from build123d import *
from build123d.topology import SkipClean

# Parameters (mm, degrees)
SKETCH_1_R               = 40
EXTRUDE_1_DEPTH          = 5
SKETCH_2_R               = 7.5
EXTRUDE_2_DEPTH          = 38
SKETCH_3_W               = 1.5
SKETCH_3_H               = 4.460741585
SKETCH_4_R               = 6
EXTRUDE_3_DEPTH          = 15
CHAMFER_1_SIZE           = 0.5
SKETCH_5_W               = 7.892485333
SKETCH_5_H               = 4
CUT_EXTRUDE_1_DEPTH      = 15
FILLET_1_R               = 2
EXTRUDE_START            = 33
SKETCH_6_R               = 40
SKETCH_6_R_2             = 30
EXTRUDE_4_DEPTH          = 33
PATTERN_CIRCULAR_1_COUNT = 4
CUT_EXTRUDE_2_DEPTH      = 33
PATTERN_CIRCULAR_2_COUNT = 2
PATTERN_CIRCULAR_2_ANGLE = 90
SKETCH_12_R              = 8.5
CUT_EXTRUDE_3_DEPTH      = 2
HOLE_WIZARD_M6_1_D       = 5
HOLE_WIZARD_M6_1_DEPTH   = 15
HOLE_WIZARD_M6_1_TIP     = 1.502151548
CUT_EXTRUDE_4_DEPTH      = 10
PATTERN_CIRCULAR_3_COUNT = 4
CHAMFER_2_SIZE           = 2
HOLE_WIZARD_M5_1_D       = 4.2
HOLE_WIZARD_M5_1_DEPTH   = 12.4
HOLE_WIZARD_M5_1_TIP     = 1.2618073


# Some blends are built 0.0001 mm under size
with BuildPart() as part:
    # 草图1 → 凸台-拉伸1 (new body)
    with BuildSketch(Plane.XY):
        with Locations((-62.277052722, 0)):
            Circle(SKETCH_1_R)
    extrude(amount=EXTRUDE_1_DEPTH)

    # 草图2 → 凸台-拉伸2 (add)
    with BuildSketch(Plane.XY.offset(5)):
        with Locations((-62.277052722, 0)):
            Circle(SKETCH_2_R)
    extrude(amount=EXTRUDE_2_DEPTH)

    # 草图3 → 切除-旋转1 (revolve, cut)
    with BuildSketch(Plane(origin=(0, 0, 0), x_dir=(0, 0, -1), z_dir=(0, -1, 0)), mode=Mode.PRIVATE) as cut_revolve_1_sk:
        with Locations((-40.75, -53.54668193)):
            Rectangle(SKETCH_3_W, SKETCH_3_H)
    revolve(cut_revolve_1_sk.sketch.rotate(Axis((-62.277052722, 0, 23.170133407), (0, 0, 1)), 180), axis=Axis((-62.277052722, 0, 23.170133407), (0, 0, 1)), mode=Mode.SUBTRACT)

    # 草图4 → 凸台-拉伸3 (add)
    with BuildSketch(Plane.XY.offset(43)):
        with Locations((-62.277052722, 0)):
            Circle(SKETCH_4_R)
    extrude(amount=EXTRUDE_3_DEPTH)

    # 倒角1
    chamfer_1_edges = [part.edges().sort_by_distance(p)[0] for p in [
        (-68.277052722, 0, 58),
        (-102.277052722, 0, 5),
        (-69.777052722, 0, 43),
    ]]
    chamfer(chamfer_1_edges, length=CHAMFER_1_SIZE)

    # 草图5 → 切除-拉伸1 (cut)
    with BuildSketch(Plane.XY.offset(58)):
        with Locations((-54.330810056, 0)):
            Rectangle(SKETCH_5_W, SKETCH_5_H)
    extrude(amount=-CUT_EXTRUDE_1_DEPTH, mode=Mode.SUBTRACT)

    # 圆角1
    fillet_1_edges = [part.edges().sort_by_distance(p)[0] for p in [
        (-57.448625597, -2, 43),
        (-57.448625597, 2, 43),
    ]]
    fillet(fillet_1_edges, radius=FILLET_1_R - 0.0001)  # a hair under: the kernel refuses the full size

    # 草图6 → 凸台-拉伸4 (add)
    with SkipClean():  # the faces are left unmerged after this step: merging them gives an invalid solid
        with BuildSketch(Plane(origin=(0, 0, 0), x_dir=(-1, 0, 0), z_dir=(0, 0, -1)).offset(EXTRUDE_START)):
            with Locations((62.277052722, 0)):
                Circle(SKETCH_6_R)
            with Locations((62.277052722, 0)):
                Circle(SKETCH_6_R_2, mode=Mode.SUBTRACT)
        extrude(amount=-EXTRUDE_4_DEPTH)

    # 草图9 → M8 螺纹孔1 (revolve, cut)
    with SkipClean():  # the faces are left unmerged after this step: merging them gives an invalid solid
        with BuildSketch(Plane(origin=(-97.277052722, 0, -33), x_dir=(0, 1, 0), z_dir=(1, 0, 0))):
            Polygon((0, 0), (0, 21.792926105), (3.4, 19.75), (3.4, 0), align=None)
        hole_wizard_m8_1 = revolve(axis=Axis((-97.277052722, 0, -39.35), (0, 0, 1)), mode=Mode.SUBTRACT)

    # 阵列(圆周)1: M8 螺纹孔1 ×4 about axis
    with SkipClean():  # the faces are left unmerged after this step: merging them gives an invalid solid
        pattern_circular_1_axis = Axis((-62.277052722, 0, 0), (0, 0, 1))
        for i in range(1, PATTERN_CIRCULAR_1_COUNT):
            add(hole_wizard_m8_1.rotate(pattern_circular_1_axis, i * 360 / PATTERN_CIRCULAR_1_COUNT), mode=Mode.SUBTRACT)

    # 草图11 → 切除-拉伸2 (cut)
    with SkipClean():  # the faces are left unmerged after this step: merging them gives an invalid solid
        with BuildSketch(Plane(origin=(0, 0, -33), x_dir=(-1, 0, 0), z_dir=(0, 0, -1))):
            Polygon((-32.267123115, 73.330972402), (135.608025124, -94.544175837), (156.82122856, -73.330972402), (-11.05391968, 94.544175837), align=None)
        cut_extrude_2 = extrude(amount=-CUT_EXTRUDE_2_DEPTH, mode=Mode.SUBTRACT)
    add(part.part.scale(1), mode=Mode.REPLACE)  # the faces are merged on a copy

    # 阵列(圆周)2: 切除-拉伸2 ×2 about axis
    pattern_circular_2_axis = Axis((-62.277052722, 0, -33), (0, 0, 1))
    for i in range(1, PATTERN_CIRCULAR_2_COUNT):
        add(cut_extrude_2.rotate(pattern_circular_2_axis, i * PATTERN_CIRCULAR_2_ANGLE / (PATTERN_CIRCULAR_2_COUNT - 1)), mode=Mode.SUBTRACT)

    # 草图12 → 切除-拉伸3 (cut)
    with BuildSketch(Plane(origin=(0, 0, 0), x_dir=(-1, 0, 0), z_dir=(0, 0, -1))):
        with Locations((62.277052722, 0)):
            Circle(SKETCH_12_R)
    extrude(amount=-CUT_EXTRUDE_3_DEPTH, mode=Mode.SUBTRACT)

    # M6 螺纹孔1
    with Locations(Plane(origin=(0, 0, 2), x_dir=(-1, 0, 0), z_dir=(0, 0, -1))):
        with Locations((62.277052722, 0)):
            Hole(HOLE_WIZARD_M6_1_D / 2, depth=HOLE_WIZARD_M6_1_DEPTH)
            with Locations((0, 0, -(HOLE_WIZARD_M6_1_DEPTH + HOLE_WIZARD_M6_1_TIP / 2))):  # 118° drill point
                Cone(0, HOLE_WIZARD_M6_1_D / 2, HOLE_WIZARD_M6_1_TIP, mode=Mode.SUBTRACT)

    # 草图15 → 切除-拉伸4 (cut)
    with BuildSketch(Plane(origin=(0, 0, 0), x_dir=(-1, 0, 0), z_dir=(0, 0, -1))):
        with BuildLine():
            Line((79.954722252, 31.819805153), (83.490256158, 35.355339059))
            ThreePointArc((83.490256158, 35.355339059), (97.632391781, 35.355339059), (97.632391781, 21.213203436))
            Line((97.632391781, 21.213203436), (94.096857875, 17.67766953))
            ThreePointArc((94.096857875, 17.67766953), (79.954722252, 17.67766953), (79.954722252, 31.819805153))
        make_face()
    cut_extrude_4 = extrude(amount=-CUT_EXTRUDE_4_DEPTH, mode=Mode.SUBTRACT)

    # 阵列(圆周)3: 切除-拉伸4 ×4 about axis
    pattern_circular_3_axis = Axis((-62.277052722, 0, 0), (0, 0, 1))
    for i in range(1, PATTERN_CIRCULAR_3_COUNT):
        add(cut_extrude_4.rotate(pattern_circular_3_axis, i * 360 / PATTERN_CIRCULAR_3_COUNT), mode=Mode.SUBTRACT)

    # 倒角2
    # the kernel refuses this chamfer: 2, 1.641704769 mm, written as the material it takes off along each edge
    with BuildSketch(Plane(origin=(-41.961992659, -34.457195687, 9.643365976), x_dir=(-0.8715539040567665, -0.4902996964341389, 0), z_dir=(0, 0, -1)), Plane(origin=(-27.819857035, 20.315060063, 9.643365976), x_dir=(0.49029969643413934, -0.8715539040567662, 0), z_dir=(0, 0, -1)), Plane(origin=(-82.592112785, 34.457195687, 9.643365976), x_dir=(0.8715539040567699, 0.4902996964341327, 0), z_dir=(0, 0, -1)), Plane(origin=(-96.734248409, -20.315060063, 9.643365976), x_dir=(-0.4902996964341341, 0.8715539040567691, 0), z_dir=(0, 0, -1))) as chamfer_2_piece_1:
        with BuildLine():
            Line((1.622634648, 0), (CHAMFER_2_SIZE * 0.269587435566, CHAMFER_2_SIZE * 0.96297591589))
            Line((CHAMFER_2_SIZE * 0.269587435566, CHAMFER_2_SIZE * 0.96297591589), (0, 0))
            ThreePointArc((0, 0), (0.83091626, -0.008223992), (1.622634648, 0))
        make_face()
    extrude(amount=14.786731952, mode=Mode.SUBTRACT)
    with BuildSketch(Plane(origin=(-27.819857035, -20.315060063, 9.643365976), x_dir=(0.49029969643413596, 0.871553904056768, 0), z_dir=(0, 0, -1)), Plane(origin=(-41.961992659, 34.457195687, 9.643365976), x_dir=(-0.8715539040567644, 0.4902996964341427, 0), z_dir=(0, 0, -1)), Plane(origin=(-96.734248409, 20.315060063, 9.643365976), x_dir=(-0.49029969643413984, -0.8715539040567659, 0), z_dir=(0, 0, -1)), Plane(origin=(-82.592112785, -34.457195687, 9.643365976), x_dir=(0.8715539040567665, -0.4902996964341389, 0), z_dir=(0, 0, -1))) as chamfer_2_piece_2:
        with BuildLine():
            Line((1.622634648, 0), (CHAMFER_2_SIZE * 0.269587435566, -CHAMFER_2_SIZE * 0.96297591589))
            Line((CHAMFER_2_SIZE * 0.269587435566, -CHAMFER_2_SIZE * 0.96297591589), (0, 0))
            ThreePointArc((0, 0), (0.83091626, 0.008223992), (1.622634648, 0))
        make_face()
    extrude(amount=14.786731952, mode=Mode.SUBTRACT)

    # M5 螺纹孔1
    with Locations(Plane.XY.offset(58)):
        with Locations((-62.277052722, 0)):
            Hole(HOLE_WIZARD_M5_1_D / 2, depth=HOLE_WIZARD_M5_1_DEPTH)
            with Locations((0, 0, -(HOLE_WIZARD_M5_1_DEPTH + HOLE_WIZARD_M5_1_TIP / 2))):  # 118° drill point
                Cone(0, HOLE_WIZARD_M5_1_D / 2, HOLE_WIZARD_M5_1_TIP, mode=Mode.SUBTRACT)


solid = part.part
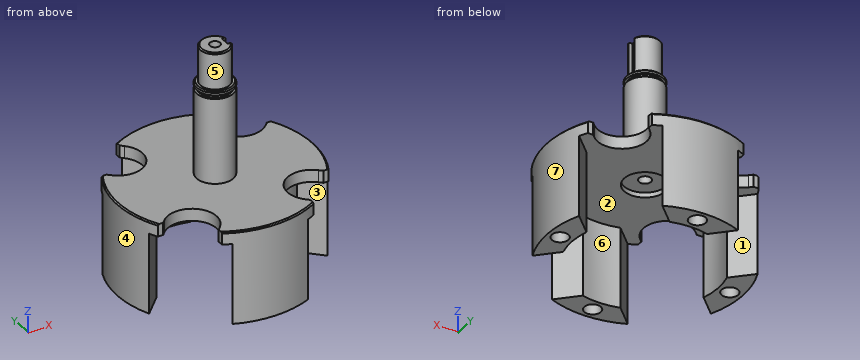
Could you check a few things on this model? Use its own coordinates, in mm. Face numbers are marked on the shaded views. A direction names the side the tool comes from. Coordinates: 2 decimals unless noted, no trailing zeros. Write each loop counter-clockwise with the first axis right and the second up, starting at its lowest first coordinate (ties: lowest second). Pieces come first, ordered by that corner, then holes. Notation, with made-up numbers: (27.5, -19) - (78.5, -19) arc R21 cw to (78.5, -2) - close; hole circle Ø8 at (51, -35.5). An arc over 180 degrees is marked (long way). Put each result on its own line as item: value. Start each with the question number.
Q1. I'm going to push flat-ended pins straight in: P1, Ø8, axis at x = -51.5, z = 23.5, coming from the -Y side; P2, Ø8, axis at x = -50, z = -12.5, coming from the -Y side; P3, Ø1.1, axis at y = -34, z = 3, coming from the -X side; P4, Ø5, axis at x = -42, z = -3.5, coming from the -Y side. Where does each tip first touch, or does it pass through?
Q2. I want a section at A-A on z = -26.5. Write out the boundary of the cut face in (x, y).
Q3. I want a section at D-D on x = -89. Write out the boundary of the cut face in (y, z), plus the area to 3 significant figures.
Q4. I want a section at C-C on z = 35. Write out the boundary of the cut face in (x, y).
Q5. Please list where these lines run through material, in increasing order: L1, parallel to Z at x = -77.5, y = -31; L2, parallel to Y at x = -79.5, z = 1; L3, parallel to X at y = 0, z = 12.
Q6. I want a section at B-B on x = -37.5. Write out the boundary of the cut face in (y, z).
Q7. Which directions (+Z, -Z, +X, -X, +Y, -Y) give clear straight access to the entire face, cutting with the end or side of a thin tool? Please do the marked faces 1, 2 and 3.
Q8. Thinking about a two-plate mould opening in X: for the marked faces 4, 5, 6 and 7, which applies, pulls with the +X half, pulls with the -X half, needs draft (parallel to the pull), parting line crosses it, or undercut?
Checks:
1. P1: y = -3.21
1. P2: y = -39.13
1. P3: x = -81.18
1. P4: through
2. outline: (-99.1, -15.61) - (-91.25, -7.76) arc R30 cw to (-91.25, 7.76) - (-99.1, 15.61) arc R40 ccw to start; (-77.89, -36.83) arc R40 ccw to (-46.66, -36.83) - (-54.51, -28.98) arc R30 cw to (-70.04, -28.98) - close; (-77.89, 36.83) - (-70.04, 28.98) arc R30 cw to (-54.51, 28.98) - (-46.66, 36.83) arc R40 ccw to start; (-33.3, -7.76) - (-25.45, -15.61) arc R40 ccw to (-25.45, 15.61) - (-33.3, 7.76) arc R30 cw to start; hole circle Ø6.8 at (-97.28, 0); hole circle Ø6.8 at (-62.28, -35); hole circle Ø6.8 at (-62.28, 35); hole circle Ø6.8 at (-27.28, 0)
3. outline: (-14.95, 0) - (14.95, 0) - (14.95, 5) - (-14.95, 5) - close
3. area: 149 mm²
4. outline: circle Ø15 at (-62.28, 0)
5. L1: 0 to 5
5. L2: -36.1 to -31.33, -18.16 to 18.16, 31.33 to 36.1
5. L3: -69.78 to -64.78, -59.78 to -54.78
6. outline: (-14.75, 0) - (14.75, 0) - (14.75, 5) - (-14.75, 5) - close
7. face 1: -Z, +Y
7. face 2: -Z
7. face 3: -Z, -Y
8. face 4: pulls with the -X half
8. face 5: parting line crosses it
8. face 6: undercut
8. face 7: pulls with the +X half
